```python
from build123d import *

# Parameters (mm, degrees)
BOSS_EXTRUDE1_DEPTH = 139
SKETCH5_R           = 7.5
CUT_EXTRUDE1_DEPTH  = 152.809090637
SKETCH6_W           = 5
SKETCH6_H           = 35
BOSS_EXTRUDE2_DEPTH = 35
SKETCH7_W           = 129
SKETCH7_H           = 35
BOSS_EXTRUDE3_DEPTH = 5


with BuildPart() as part:
    # Sketch3 → Boss-Extrude1 (new body)
    with BuildSketch(Plane(origin=(0, 0, 0), x_dir=(0, 0, -1), z_dir=(1, 0, 0))):
        Polygon((-27.8080918, 35), (-27.8080918, 10), (2.1919082, 10), (2.1919082, 35), (12.1919082, 35), (12.1919082, 0), (47.1919082, 0), (47.1919082, -10), (2.1919082, -10), (2.1919082, 0), (-37.8080918, 0), (-37.8080918, 35), align=None)
    extrude(amount=BOSS_EXTRUDE1_DEPTH)

    # Sketch5 → Cut-Extrude1 (cut, through all)
    with BuildSketch(Plane(origin=(0, 0, -12.1919082), x_dir=(-1, 0, 0), z_dir=(0, 0, -1))):
        with Locations(Location((-119, 20, 0), (0, 0, 90))):
            Circle(SKETCH5_R)
        with BuildLine():
            Line((-85, 27.5), (-15, 27.5))
            ThreePointArc((-15, 27.5), (-7.5, 20), (-15, 12.5))
            Line((-15, 12.5), (-85, 12.5))
            ThreePointArc((-85, 12.5), (-92.5, 20), (-85, 27.5))
        make_face()
    extrude(amount=-CUT_EXTRUDE1_DEPTH, mode=Mode.SUBTRACT)

    # Sketch6 → Boss-Extrude2 (add)
    with BuildSketch(Plane(origin=(0, 0, 0), x_dir=(1, 0, 0), z_dir=(0, 1, 0))):
        with Locations((2.5, 29.6919082)):
            Rectangle(SKETCH6_W, SKETCH6_H)
        with Locations((136.5, 29.6919082)):
            Rectangle(SKETCH6_W, SKETCH6_H)
    extrude(amount=BOSS_EXTRUDE2_DEPTH)

    # Sketch7 → Boss-Extrude3 (add)
    with BuildSketch(Plane(origin=(0, 0, -12.1919082), x_dir=(-1, 0, 0), z_dir=(0, 0, -1))):
        with Locations((-69.5, 17.5)):
            Rectangle(SKETCH7_W, SKETCH7_H)
    extrude(amount=BOSS_EXTRUDE3_DEPTH)


solid = part.part
```
Read the model definition and answer for the solid it produces. Units are mm, in the model's axes. A direction names the side the tool comes from. Coordinates: 2 decimals unless noted, no trailing zeros. Loops run counter-clockwise (first coordinate to the right, second up) from the corner with the lowest first, then second, coordinate; pieces in that order, holes last. Notation, with made-up numbers: (63, -20.5) -> (102, -20.5) arc R26 ccw to (102, -2.5) -> close; hole circle Ø11 at (40, -7). An arc over 180 degrees is marked (long way). Return JSON: item names as keys, results as strings.
Item 1: Flat-ended cylindrical pins translate along their axes: P1, Ø15, axis at x = 92.5, z = -36, coming from the +Y side; P2, Ø3, axis at x = 53.5, z = 2.5, coming from the -Y side; P3, Ø10, axis at x = 90.5, y = 7.5, coming from the -Z side. Find the tip coordinate at first contact, or state that the pin passes through.
Answers:
{"P1": "stops at y = 0", "P2": "stops at y = 0", "P3": "stops at z = -17.19"}
Item 2: Find section B-B (z = -5). Determine the outline of the cut face in (x, y).
Answers:
{"outline": "(0, -10) -> (139, -10) -> (139, 35) -> (0, 35) -> close; hole (15, 12.5) -> (85, 12.5) arc R7.5 ccw to (85, 27.5) -> (15, 27.5) arc R7.5 ccw to start; hole circle Ø15 at (119, 20)"}
Item 3: For a pull along X with two mould halves and no side action, classify faces 4 (the flat face through (139, 13, -15)), 5 (the flat face through (134, 17, -32)), 6 (the flat face through (0, 12, -14)), 7 (the cylindrical face through (111.68, 18.37, 32.74)) as +X half, -X half, draft (parallel to the pull), parting line (faces both ways), or undercut.
Answers:
{"face 4": "+X half", "face 5": "undercut", "face 6": "-X half", "face 7": "undercut"}
Item 4: Find section C-C (x = 119). Determine the outline of the cut face in (y, z), plus the area to 4 significant figures.
Answers:
{"outline": "(-10, -47.19) -> (0, -47.19) -> (0, -17.19) -> (35, -17.19) -> (35, -2.19) -> (27.5, -2.19) -> (27.5, -12.19) -> (12.5, -12.19) -> (12.5, -2.19) -> (10, -2.19) -> (10, 27.81) -> (12.5, 27.81) -> (12.5, 37.81) -> (0, 37.81) -> (0, -2.19) -> (-10, -2.19) -> close; (27.5, 27.81) -> (35, 27.81) -> (35, 37.81) -> (27.5, 37.81) -> close", "area": "1,325 mm2"}
Item 5: For faces 1 (the flat face through (69, 0, 18)), 2 (the flat face through (69, 0, -32)), 3 (the flat face through (119, 20, -12.192)), determine the directions among +Z, -Z, +X, -X, +Y, -Y from which every point of the face is accessible in a straight line to the end or side of a thin tool.
Answers:
{"face 1": "+Z, +X, -X, -Y", "face 2": "-Z, +Y", "face 3": "+Z"}
Item 6: Find section D-D (y = 2.5). Determine the outline of the cut face in (x, z), plus the area to 4 significant figures.
Answers:
{"outline": "(0, -47.19) -> (5, -47.19) -> (5, -17.19) -> (134, -17.19) -> (134, -47.19) -> (139, -47.19) -> (139, 37.81) -> (0, 37.81) -> close", "area": "7,945 mm2"}
Item 7: Find the intervals of material crossed by probe 1 along X at (y, z) = (20, -7.75); probe 2 along Z at (x, y) = (48, 11.5); probe 3 along X at (y, z) = (26, -25), in increasing order.
Answers:
{"probe 1": "x = 0 to 7.5, 92.5 to 111.5, 126.5 to 139", "probe 2": "z = -17.19 to -2.19, 27.81 to 37.81", "probe 3": "x = 0 to 5, 134 to 139"}
Item 8: Find section A-A (y = 20). Determine the outline of the cut face in (x, z).
Answers:
{"outline": "(0, -47.19) -> (5, -47.19) -> (5, -17.19) -> (134, -17.19) -> (134, -47.19) -> (139, -47.19) -> (139, -2.19) -> (126.5, -2.19) -> (126.5, -12.19) -> (111.5, -12.19) -> (111.5, -2.19) -> (92.5, -2.19) -> (92.5, -12.19) -> (7.5, -12.19) -> (7.5, -2.19) -> (0, -2.19) -> close; (0, 27.81) -> (7.5, 27.81) -> (7.5, 37.81) -> (0, 37.81) -> close; (92.5, 27.81) -> (111.5, 27.81) -> (111.5, 37.81) -> (92.5, 37.81) -> close; (126.5, 27.81) -> (139, 27.81) -> (139, 37.81) -> (126.5, 37.81) -> close"}
